from build123d import *

# Parameters (mm, degrees)
F0_R     = 39.060961
F0_R_2   = 17.961564
F1_DEPTH = 25.4
F3_DEPTH = 12.7


with BuildPart() as f1:
    # F0 (on Front) → F1 (new body)
    with BuildSketch(Plane.XZ):
        Circle(F0_R)
        Circle(F0_R_2, mode=Mode.SUBTRACT)
    extrude(amount=F1_DEPTH)

    # F2 (on Front) → F3 (join)
    with BuildSketch(Plane.XZ):
        with BuildLine():
            Line((-5.171036, 58.106368), (-31.56358, 23.489174))
            Line((-31.56358, 23.489174), (30.095503, 23.489174))
            Line((30.095503, 23.489174), (5.014983, 57.990182))
            ThreePointArc((5.014983, 57.990182), (-0.048852, 60.605962), (-5.171036, 58.106368))
        make_face()
    extrude(amount=F3_DEPTH)


solid = f1.part
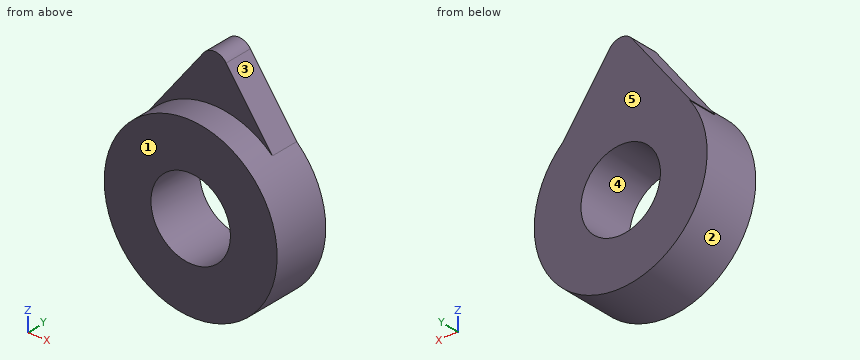
Design review of the part built by this model. Coordinates are the model's own, in mm. Face numbers are marked on the shaded views. A direction names the side the tool comes from. Round coordinates to 2 decimals unless told otherwise and drop trailing zeros. Write each loop counter-clockwise with the first axis right and the second up, starting at its lowest first coordinate (ties: lowest second). Pieces come first, ordered by that corner, then holes.
Item 1: For the marked faces 1 and 2, list the 3-axis set-ups (+Z, -Z, +X, -X, +Y, -Y) from which the entire face can be reached by the end or side of a thin tool; tool diameter is ignored.
Item 2: Consider section D-D on x = 11.5. Give the boundary of the cut face in (y, z), and give its area (3 significant figures).
Item 3: Consider section C-C on y = -20. Give the boundary of the cut face in (x, z).
Item 4: For pin 1 Ø1.5 at (y, z) = (-18.5, -0.5) entering from +X; pin 2 Ø3 at (x, y) = (-29, -22) entering from +Z; pin 3 Ø5 at (x, y) = (-8, -6.5) entering from +Z; pin 4 Ø3 at (x, y) = (-14.5, -16.5) entering from -Z, all flat-tipped, find the tip position at first contact; note any pin that passes through.
Item 5: Wall thickness on L1, parallel to Z at x = 0, y = -13.5; L2, parallel to Z at x = 0, y = -12; L3, parallel to X at y = -21, z = -9: over which ranges is each line inside the solid? List them lowest first.
Item 6: Draft analysis for pull direction Z (two halves, no side actions). For the marked faces 3, 4 and 5, state which applies: released by +Z, released by -Z, zero draft, split by the parting line, or undercut.
Item 7: Consider section B-B on x = -9. Give the boundary of the cut face in (y, z).
Item 8: Consider section A-A on z = 0. Give the boundary of the cut face in (x, y), and give its area (3 significant figures).
Check values:
1. face 1: +Z, -Z, +X, -X, -Y
1. face 2: -Y
2. outline: (-25.4, -37.33) - (0, -37.33) - (0, -13.8) - (-25.4, -13.8) - close; (-25.4, 13.8) - (0, 13.8) - (0, 49.07) - (-12.7, 49.07) - (-12.7, 37.33) - (-25.4, 37.33) - close
2. area: 1,340 mm2
3. outline: circle Ø78.12 at (0, 0); hole circle Ø35.92 at (0, 0)
4. pin 1: stops at x = 39.06
4. pin 2: stops at z = 27.74
4. pin 3: stops at z = 57.67
4. pin 4: stops at z = -36.83
5. L1: z = -39.06 to -17.96, 17.96 to 39.06
5. L2: z = -39.06 to -17.96, 17.96 to 60.61
5. L3: x = -38.01 to -15.54, 15.54 to 38.01
6. face 3: released by +Z
6. face 4: undercut
6. face 5: zero draft
7. outline: (-25.4, -38.01) - (0, -38.01) - (0, -15.54) - (-25.4, -15.54) - close; (-25.4, 15.54) - (0, 15.54) - (0, 53.08) - (-12.7, 53.08) - (-12.7, 38.01) - (-25.4, 38.01) - close
8. outline: (-39.06, -25.4) - (-17.96, -25.4) - (-17.96, 0) - (-39.06, 0) - close; (17.96, -25.4) - (39.06, -25.4) - (39.06, 0) - (17.96, 0) - close
8. area: 1,070 mm2
